For this review, use the dimensioned drawing (mm, ordinates from the lowest corner) and the shaded views. A direction names the side the tool comes from. Coordinates: 2 decimals unless noted, no trailing zeros. Order: outer loops, then holes, each group sorted by start corner. A loop starts at its lowest first (then second) coordinate and runs counter-clockwise, first axis right, second up. Notation, with made-up numbers: (63.25, -31) -> (70.25, -31) arc R24 cw to (70.25, -10) -> close; hole circle Ø3 at (55, 17.5). An arc over 180 degrees is marked (long way). Return JSON: item names as keys, results as strings. Group by question number.
Item 1: Take a section at B-B (x = 58). Write out the cut boundary in (y, z), then the cut area to 3 significant figures.
Item 2: Take a section at D-D (x = 33). Write out the cut boundary in (y, z), then the cut area to 3 significant figures.
Item 3: Take a section at A-A (y = 50). Write out the cut boundary in (x, z), then the cut area to 3 significant figures.
Item 4: For line 1 along Y through (x, z) = (95, 22.4); line 2 along Y through (x, z) = (50, 12.5); line 3 along X through (y, z) = (49, 8.75), list the stretches that pass through material, from the lowest coordinate up.
Item 5: Insertion check: pin 1 (4 mm diameter, centred on y = 6.5, z = 21.5, fed in from -X); pin 2 (6.5 mm diameter, centred on x = 95, y = 50, fed in from -Z); pin 3 (1 mm diameter, centred on x = 43.5, z = 13, fed in from +Y). Each pin has a flat end and moves straight along its axis. Give the tip position at first contact, or say it passes through.
Item 6: Machinability: for the marked faces 4 and 5, which of the approach directions +Z, -Z, +X, -X, +Y, -Y give a long, thin tool a straight path to every point of the face, cutting with its end or side? Answer none if there is none.
Item 7: Draft analysis for pull direction X (two halves, no side actions). For the marked faces 1, 2 and 3, state which applies: +X half, -X half, draft (parallel to the pull), parting line (faces both ways), or undercut.
Item 8: Take a section at C-C (z = 15). Write out the cut boundary in (x, y), then the cut area to 3 significant figures.
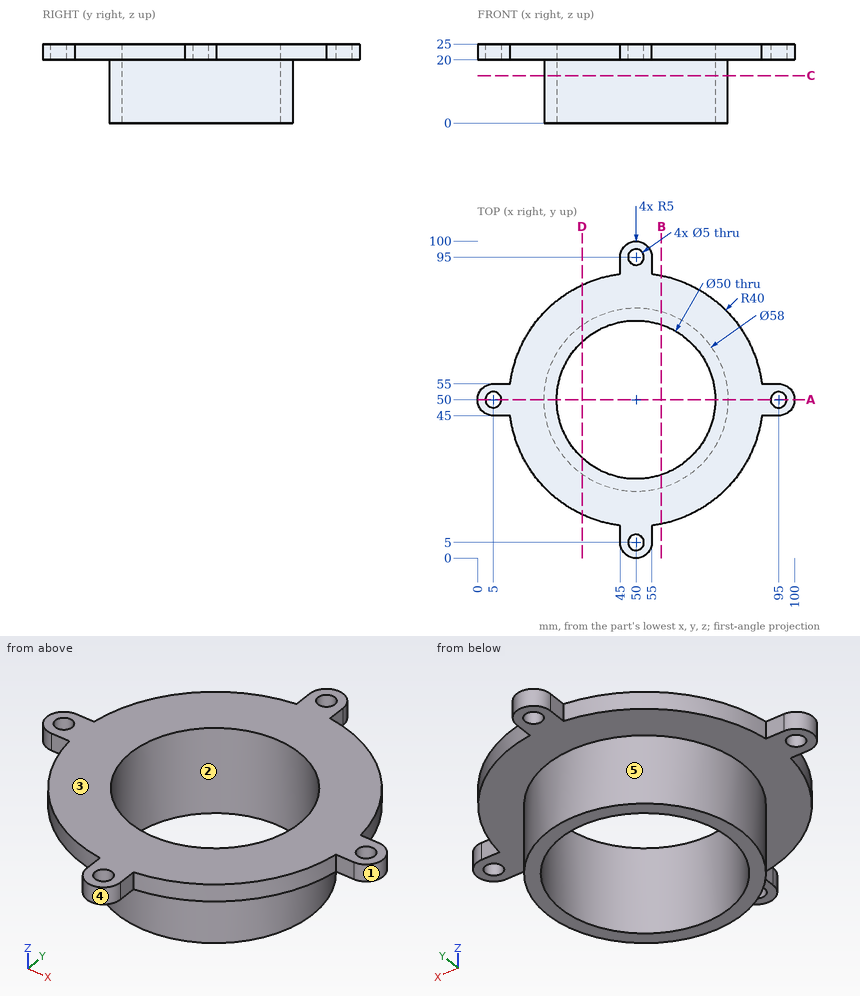
Findings below:
{
 "1": {"outline": "(10.81, 20) -> (22.13, 20) -> (22.13, 0) -> (26.31, 0) -> (26.31, 25) -> (10.81, 25) -> close; (73.69, 0) -> (77.87, 0) -> (77.87, 20) -> (89.19, 20) -> (89.19, 25) -> (73.69, 25) -> close", "area": "323 mm2"},
 "2": {"outline": "(13.79, 20) -> (26.51, 20) -> (26.51, 0) -> (31.67, 0) -> (31.67, 25) -> (13.79, 25) -> close; (68.33, 0) -> (73.49, 0) -> (73.49, 20) -> (86.21, 20) -> (86.21, 25) -> (68.33, 25) -> close", "area": "385 mm2"},
 "3": {"outline": "(0, 20) -> (2.5, 20) -> (2.5, 25) -> (0, 25) -> close; (7.5, 20) -> (21, 20) -> (21, 0) -> (25, 0) -> (25, 25) -> (7.5, 25) -> close; (75, 0) -> (79, 0) -> (79, 20) -> (92.5, 20) -> (92.5, 25) -> (75, 25) -> close; (97.5, 20) -> (100, 20) -> (100, 25) -> (97.5, 25) -> close", "area": "360 mm2"},
 "4": {"line 1": "y = 45 to 47.5, 52.5 to 55", "line 2": "y = 21 to 25, 75 to 79", "line 3": "x = 21.02 to 25.02, 74.98 to 78.98"},
 "5": {"pin 1": "stops at x = 45", "pin 2": "stops at z = 20", "pin 3": "stops at y = 78.37"},
 "6": {"face 4": "+Z, -Z, -Y", "face 5": "-Z"},
 "7": {"face 1": "+X half", "face 2": "undercut", "face 3": "draft"},
 "8": {"outline": "circle Ø58 at (50, 50); hole circle Ø50 at (50, 50)", "area": "679 mm2"}
}
